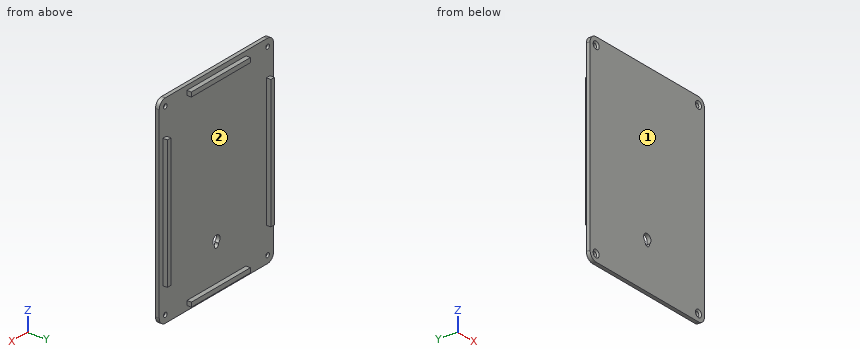
```python
from build123d import *

# Parameters (mm, degrees)
EXTRUDE_1_DEPTH     = 2.5
SKETCH_2_R          = 1.5
CUT_EXTRUDE_1_DEPTH = 11
SKETCH_3_W          = 49
SKETCH_3_H          = 3
SKETCH_3_W_2        = 3
SKETCH_3_H_2        = 87
EXTRUDE_2_DEPTH     = 3
CUT_EXTRUDE_2_DEPTH = 6
CHAMFER_1_SIZE      = 1


with BuildPart() as part:
    # Эскиз1 → Бобышка-Вытянуть1 (new body)
    with BuildSketch(Plane(origin=(0, 0, 0), x_dir=(1, 0, 0), z_dir=(0, 1, 0))):
        with BuildLine():
            Line((-42.5, -66.5), (42.5, -66.5))
            ThreePointArc((42.5, -66.5), (46.035533906, -65.035533906), (47.5, -61.5))
            Line((47.5, -61.5), (47.5, 61.5))
            ThreePointArc((47.5, 61.5), (46.035533906, 65.035533906), (42.5, 66.5))
            Line((42.5, 66.5), (-42.5, 66.5))
            ThreePointArc((-42.5, 66.5), (-46.035533906, 65.035533906), (-47.5, 61.5))
            Line((-47.5, 61.5), (-47.5, -61.5))
            ThreePointArc((-47.5, -61.5), (-46.035533906, -65.035533906), (-42.5, -66.5))
        make_face()
    extrude(amount=EXTRUDE_1_DEPTH)

    # Эскиз2 → Вырез-Вытянуть1 (cut)
    with BuildSketch(Plane(origin=(0, 2.5, 0), x_dir=(1, 0, 0), z_dir=(0, 1, 0))):
        with Locations((-42.5, 61.5)):
            Circle(SKETCH_2_R)
        with Locations((42.5, 61.5)):
            Circle(SKETCH_2_R)
        with Locations((42.5, -61.5)):
            Circle(SKETCH_2_R)
        with Locations((-42.5, -61.5)):
            Circle(SKETCH_2_R)
    extrude(amount=-CUT_EXTRUDE_1_DEPTH, mode=Mode.SUBTRACT)

    # Эскиз3 → Бобышка-Вытянуть2 (add)
    with BuildSketch(Plane(origin=(0, 2.5, 0), x_dir=(1, 0, 0), z_dir=(0, 1, 0))):
        with Locations((0, 62)):
            Rectangle(SKETCH_3_W, SKETCH_3_H)
        with Locations((0, -62)):
            Rectangle(SKETCH_3_W, SKETCH_3_H)
        with Locations((-43, 0)):
            Rectangle(SKETCH_3_W_2, SKETCH_3_H_2)
        with Locations((43, 0)):
            Rectangle(SKETCH_3_W_2, SKETCH_3_H_2)
    extrude(amount=EXTRUDE_2_DEPTH)

    # Эскиз4 → Вырез-Вытянуть2 (cut)
    with BuildSketch(Plane(origin=(0, 2.5, 0), x_dir=(1, 0, 0), z_dir=(0, 1, 0))):
        with BuildLine():
            ThreePointArc((-1.673910041, 37.489583333), (0, 39.75), (1.673910041, 37.489583333))
            ThreePointArc((1.673910041, 37.489583333), (0, 32), (-1.673910041, 37.489583333))
        make_face()
    extrude(amount=-CUT_EXTRUDE_2_DEPTH, mode=Mode.SUBTRACT)

    # Фаска1
    chamfer_1_edges = [part.edges().sort_by_distance(p)[0] for p in [
        (-44, 0, 61.5),
        (41, 0, 61.5),
        (41, 0, -61.5),
        (-44, 0, -61.5),
    ]]
    chamfer(chamfer_1_edges, length=CHAMFER_1_SIZE)


solid = part.part
```
Model file for the job. Use its own axes, mm. Face numbers are marked on the shaded views. Round coordinates to 2 decimals unless told otherwise and drop trailing zeros. Order: outer loops, then holes, each group sorted by start corner. A loop starts at its lowest first (then second) coordinate and runs counter-clockwise, first axis right, second up. Notation, with made-up numbers: M 34,63 L 54,63 A12 cw 54,81 Z; hole C 76.25,2.25 d11. An arc over 180 degrees is marked long. Use CSV: the item, a comma, the result in double quotes.
Item 1: Pull direction X, two halves, no side cores. Call the marked faces 1 and 2: released by +X, released by -X, zero draft, split by the parting line, or undercut.
Worked answers:
face 1,"zero draft"
face 2,"undercut"
Item 2: Saw through at A-A (y = 4.6). List the corners of the cut face in (x, z), plus the area to 3 significant figures.
Worked answers:
outline,"M -44.5,-43.5 L -41.5,-43.5 L -41.5,43.5 L -44.5,43.5 Z; M -24.5,-63.5 L 24.5,-63.5 L 24.5,-60.5 L -24.5,-60.5 Z; M -24.5,60.5 L 24.5,60.5 L 24.5,63.5 L -24.5,63.5 Z; M 41.5,-43.5 L 44.5,-43.5 L 44.5,43.5 L 41.5,43.5 Z"
area,"816 mm²"
Item 3: Probe probe 1 along X at (y, z) = (2.05, -61.5); probe 2 along Z at (x, y) = (-42.5, 1.8); probe 3 along Z at (x, y) = (-6.5, 2.9). List the from-to ranges inside material, lowest first.
Worked answers:
probe 1,"-47.5 to -44, -41 to 41, 44 to 47.5"
probe 2,"-66.5 to -63, -60 to 60, 63 to 66.5"
probe 3,"-63.5 to -60.5, 60.5 to 63.5"
Item 4: Saw through at D-D (z = 26). List the corners of the cut face in (x, y), plus the area to 4 significant figures.
Worked answers:
outline,"M -47.5,0 L 47.5,0 L 47.5,2.5 L 44.5,2.5 L 44.5,5.5 L 41.5,5.5 L 41.5,2.5 L -41.5,2.5 L -41.5,5.5 L -44.5,5.5 L -44.5,2.5 L -47.5,2.5 Z"
area,"255.5 mm²"
Item 5: Saw through at C-C (z = -35). List the corners of the cut face in (x, y), plus the area to 4 significant figures.
Worked answers:
outline,"M -47.5,0 L -3,0 L -3,2.5 L -41.5,2.5 L -41.5,5.5 L -44.5,5.5 L -44.5,2.5 L -47.5,2.5 Z; M 3,0 L 47.5,0 L 47.5,2.5 L 44.5,2.5 L 44.5,5.5 L 41.5,5.5 L 41.5,2.5 L 3,2.5 Z"
area,"240.5 mm²"
Item 6: Saw through at B-B (x = 0). List the corners of the cut face in (y, z).
Worked answers:
outline,"M 0,-66.5 L 2.5,-66.5 L 2.5,-63.5 L 5.5,-63.5 L 5.5,-60.5 L 2.5,-60.5 L 2.5,-39.75 L 0,-39.75 Z; M 0,-32 L 2.5,-32 L 2.5,60.5 L 5.5,60.5 L 5.5,63.5 L 2.5,63.5 L 2.5,66.5 L 0,66.5 Z"
Item 7: Pin check, flat tips, straight feed: pin 1 (1.5 mm diameter, centred on x = -1.5, y = 3.5, fed in from -Z); pin 2 (5.5 mm diameter, centred on x = 0, z = -35, fed in from +Y); pin 3 (2.5 mm diameter, centred on y = 4, z = 9, fed in from -X); pin 4 (1.5 mm diameter, centred on x = -43.5, y = 4.5, fed in from +Z). Stop position of each tip, or through.
Worked answers:
pin 1,"z = -63.5"
pin 2,"through"
pin 3,"x = -44.5"
pin 4,"z = 43.5"
